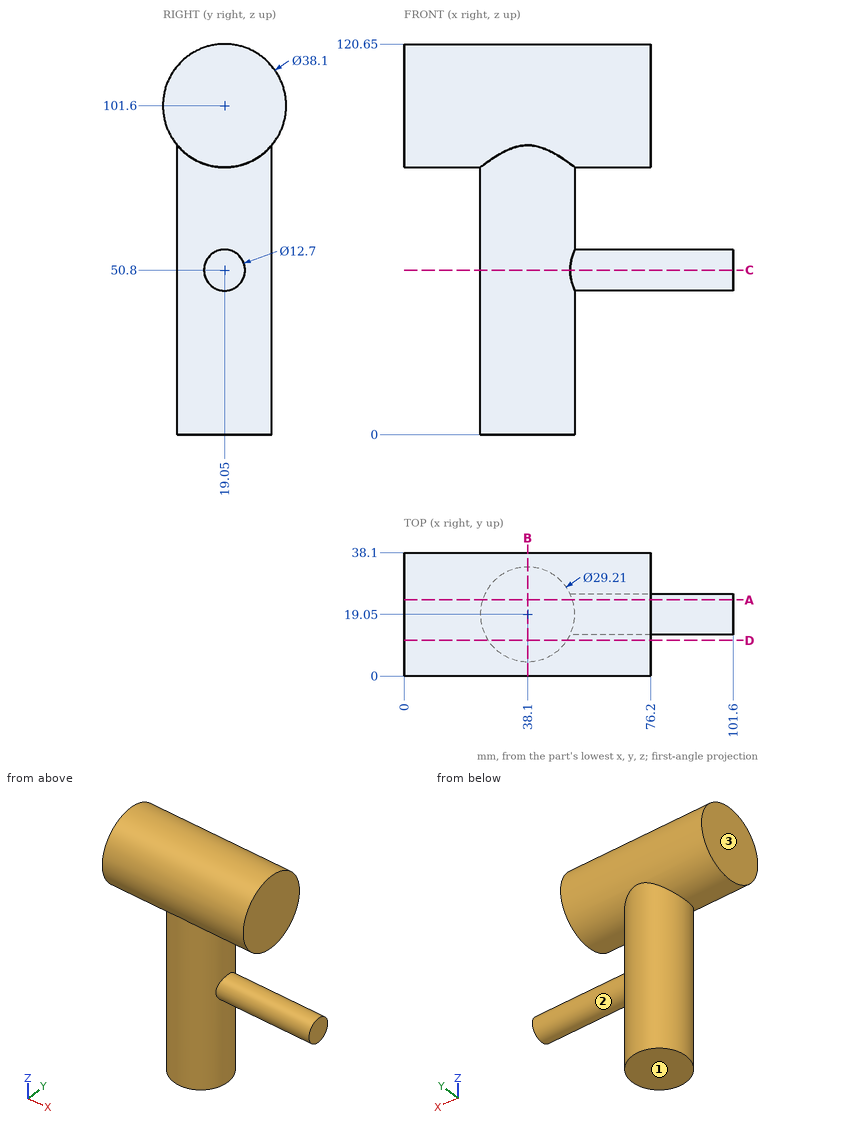
Print and shaded views of the part. All mm, measured from the part's lowest x, y and z. Give positions to 0.01 mm unless a question says otherwise; leave off trailing zeros. Loops run counter-clockwise (first coordinate to the right, second up) from the corner with the lowest first, then second, coordinate; pieces in that order, holes last. Notation, with made-up numbers: (77.5, 49.5) - (123.5, 49.5) arc R18 ccw to (123.5, 79.5) - close; hole circle Ø10 at (-3, 46.25). An arc over 180 degrees is marked (long way). One line per item, written item: value. Start each with the question number.
1. Slice it at A-A (y = 23.5). List the corners of the cut face in (x, z).
2. Pull direction Z, two halves, no side cores. Call the marked faces 1, 2 and 3: pulls with the +Z half, pulls with the -Z half, needs draft (parallel to the pull), parting line crosses it, or undercut.
3. Slice it at D-D (y = 11). List the corners of the cut face in (x, z).
4. Pin check, flat tips, straight feed: pin 1 (1.5 mm diameter, centred on x = 27, y = 28, fed in from +Z); pin 2 (1 mm diameter, centred on y = 5, z = 65.5, fed in from -X); pin 3 (1.5 mm diameter, centred on y = 13, z = 59.5, fed in from +X). Stop position of each tip, or through.
5. Probe L1, parallel to X at y = 20, z = 5; L2, parallel to X at y = 15, z = 93; L3, parallel to Z at x = 5.5, y = 7. List the from-to ranges inside material, lowest first. Write a range as from..to.
6. Slice it at C-C (z = 50.8). List the corners of the cut face in (x, y) (3 decimals).
7. Slice it at B-B (x = 38.1). List the corners of the cut face in (y, z) (3 decimals), plus the area to 3 significant figures.
Solution:
1. outline: (0, 83.08) - (24.19, 83.08) - (24.19, 0) - (52.01, 0) - (52.01, 46.27) - (101.6, 46.27) - (101.6, 55.33) - (52.01, 55.33) - (52.01, 83.08) - (76.2, 83.08) - (76.2, 120.12) - (0, 120.12) - close
2. face 1: pulls with the -Z half
2. face 2: undercut
2. face 3: needs draft
3. outline: (0, 84.33) - (25.91, 84.33) - (25.91, 0) - (50.29, 0) - (50.29, 84.33) - (76.2, 84.33) - (76.2, 118.87) - (0, 118.87) - close
4. pin 1: stops at z = 118.79
4. pin 2: stops at x = 32.65
4. pin 3: stops at x = 51.71
5. L1: x = 23.53..52.67
5. L2: x = 0..76.2
5. L3: z = 86.85..116.35
6. outline: (51.252, 12.7) - (101.6, 12.7) - (101.6, 25.4) - (51.252, 25.4) arc R14.605 ccw (long way) to start
7. outline: (4.445, 0) - (33.655, 0) - (33.655, 89.369) arc R19.05 ccw (long way) to (4.445, 89.369) - close
7. area: 3,610 mm^2
